```python
from build123d import *

# Parameters (mm, degrees)
F1_DEPTH = 6.35
F2_W     = 13.0048
F2_H     = 13.0048
F3_DEPTH = 6.351
F4_R     = 19.04999


# Not quite as in the source:
# - a fillet or chamfer is up to 0.001 mm smaller than in the source, because OpenCascade refuses the exact size


with BuildPart() as f1:
    # F0 (on Front) → F1 (new body)
    with BuildSketch(Plane.XZ):
        Polygon((0, 57.15), (0, 0), (82.55, 0), (82.55, 19.05), (19.05, 19.05), (19.05, 57.15), (215.9, 57.15), (215.9, 69.85), (47.625, 104.775), (25.4, 104.775), align=None)
    extrude(amount=F1_DEPTH)

    # F2 (on face) → F3 (cut, through all)
    with BuildSketch(Plane.XZ.offset(6.35)):
        with Locations((38.2524, 89.0524)):
            Rectangle(F2_W, F2_H)
    extrude(amount=-F3_DEPTH, mode=Mode.SUBTRACT)

    # F4 (radius 19.05 in the source; OpenCascade refuses exactly that, so slightly less here)
    f4_edges = [f1.edges().sort_by_distance(p)[0] for p in [
        (0, -3.175, 0),
        (82.55, -3.175, 0),
        (0, -3.175, 57.15),
        (47.625, -3.175, 104.775),
    ]]
    fillet(f4_edges, radius=F4_R)


solid = f1.part
```
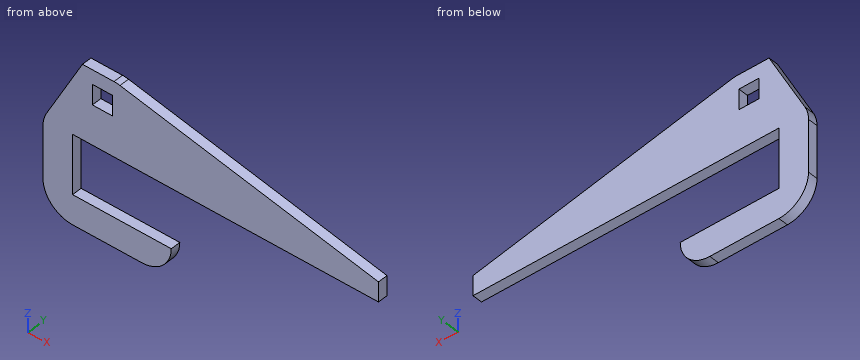
Build history of the part. All positions in model axes, mm. Round coordinates to 2 decimals unless told otherwise and drop trailing zeros. Loops run counter-clockwise (first coordinate to the right, second up) from the corner with the lowest first, then second, coordinate; pieces in that order, holes last.
Item 1: Saw through at D-D (x = 14). List the corners of the cut face in (y, z).
Item 2: Saw through at C-C (z = 24). List the corners of the cut face in (x, y).
Item 3: Saw through at A-A (x = 38). List the corners of the cut face in (y, z) (3 decimals), then the cut area to 3 significant figures.
Item 4: Drill centre lines: line 1 along Z through (x, y) = (35, -1.5) (3 decimals); line 2 along Z through (x, y) = (78.5, -1); line 3 along Z through (x, y) = (71.5, -4.5). Where is each one in solid material? Low to high.
Item 5: Pin check, flat tips, straight feed: P1, Ø1.9, axis at y = -2, z = 32.5, coming from the +X side; P2, Ø3, axis at x = 72.5, y = -2.5, coming from the -Z side. Stop position of each tip, or through.
Worked answers:
1. outline: (-6.35, 0.68) - (0, 0.68) - (0, 83.4) - (-6.35, 83.4) - close
2. outline: (0, -6.35) - (19.05, -6.35) - (19.05, 0) - (0, 0) - close
3. outline: (-6.35, 0) - (0, 0) - (0, 19.05) - (-6.35, 19.05) - close; (-6.35, 57.15) - (0, 57.15) - (0, 82.55) - (-6.35, 82.55) - close; (-6.35, 95.555) - (0, 95.555) - (0, 104.775) - (-6.35, 104.775) - close
3. area: 341 mm2
4. line 1: z = 0 to 19.05, 57.15 to 82.55, 95.555 to 104.775
4. line 2: z = 7.31 to 19.05, 57.15 to 98.37
4. line 3: z = 1.76 to 19.05, 57.15 to 99.82
5. P1: stops at x = 19.05
5. P2: stops at z = 1.54
